Design review of the part built by this model. Coordinates are the model's own, in mm. Face numbers are marked on the shaded views. A direction names the side the tool comes from. Coordinates: 2 decimals unless noted, no trailing zeros. Loops run counter-clockwise (first coordinate to the right, second up) from the corner with the lowest first, then second, coordinate; pieces in that order, holes last. Notation, with made-up numbers: (43.25, -25.75) -> (87.25, -25.75) arc R23 cw to (87.25, 1.25) -> close; hole circle Ø8 at (7, 69.25). An arc over 180 degrees is marked (long way). Use one line per item in the form item = value. Start each with the question number.
1. Machinability: for the marked faces 1, 2, 3, 4 and 5, which of the approach directions +Z, -Z, +X, -X, +Y, -Y give a long, thin tool a straight path to every point of the face, cutting with its end or side? Answer none if there is none.
2. Consider section A-A (x = 51.75). State the section outline as (y, z) points.
3. The part is to be moulded in two halves that separate along Y. For the marked faces 6, 7 and 8, say which applies: released by +Y, released by -Y, zero draft, split by the parting line, or undercut.
4. For pin 1 (3.5 mm diameter, centred on y = 9.5, z = 30.09, fed in from +X); pin 2 (1.8 mm diameter, centred on y = 8, z = 0.5, fed in from +X); pin 3 (5 mm diameter, centred on y = 8.5, z = 32, fed in from +X), all flat-tipped, find the tip position at first contact; note any pin that passes through.
5. Consider section D-D (z = 13). State the section outline as (x, y) points, then the cut area to 3 significant figures.
6. Wall thickness on line 1 (Y direction, x = 55.5, z = 23); line 2 (Z direction, x = 40.5, y = 11.25); line 3 (X direction, y = 3.25, z = 16): over which ranges is each line inside the solid? List them lowest first. Write a range as from..to.
7. Consider section C-C (z = 29). State the section outline as (x, y) points.
8. Consider section B-B (y = 9.5). State the section outline as (x, z) points, then the cut area to 3 significant figures.
from build123d import *

# Parameters (mm, degrees)
SKETCH1_W           = 26
SKETCH1_H           = 37.2
BOSS_EXTRUDE1_DEPTH = 19
SKETCH2_W           = 20
SKETCH2_H           = 10
CUT_EXTRUDE1_DEPTH  = 77.929109018
SKETCH3_R           = 1.6
CUT_EXTRUDE2_DEPTH  = 76.699707134
CUT_EXTRUDE3_DEPTH  = 76.699707134
SKETCH7_W           = 22.2
SKETCH7_H           = 10
CUT_EXTRUDE6_DEPTH  = 45.240228818
SKETCH8_R           = 1.6
CUT_EXTRUDE7_DEPTH  = 45.240228818
CHAMFER1_SIZE       = 2
SKETCH9_R           = 2.9
CUT_EXTRUDE12_DEPTH = 2


with BuildPart() as part:
    # Sketch1 → Boss-Extrude1 (new body)
    with BuildSketch(Plane(origin=(0, 0, 0), x_dir=(1, 0, 0), z_dir=(0, 1, 0))):
        with Locations((51.600679674, -15.986093244)):
            Rectangle(SKETCH1_W, SKETCH1_H)
    extrude(amount=BOSS_EXTRUDE1_DEPTH)

    # Sketch2 → Cut-Extrude1 (cut, through all)
    with BuildSketch(Plane.XY.offset(34.586093244)):
        with Locations((54.600679674, 9.5)):
            Rectangle(SKETCH2_W, SKETCH2_H)
    extrude(amount=-CUT_EXTRUDE1_DEPTH, mode=Mode.SUBTRACT)

    # Sketch3 → Cut-Extrude2 (cut, through all)
    with BuildSketch(Plane.XZ):
        with Locations(Location((55.600679674, 15.986093244, 0), (0, 0, 270))):
            Circle(SKETCH3_R)
    extrude(amount=-CUT_EXTRUDE2_DEPTH, mode=Mode.SUBTRACT)

    # Sketch4 → Cut-Extrude3 (cut, through all)
    with BuildSketch(Plane.XZ):
        Polygon((64.600679674, 24.586093244), (54.600679674, 34.586093244), (64.600679674, 34.586093244), align=None)
        Polygon((64.600679674, 7.386093244), (54.600679674, -2.613906756), (64.600679674, -2.613906756), align=None)
    extrude(amount=-CUT_EXTRUDE3_DEPTH, mode=Mode.SUBTRACT)

    # Sketch7 → Cut-Extrude6 (cut, through all)
    with BuildSketch(Plane(origin=(44.600679674, 0, 0), x_dir=(0, 0, -1), z_dir=(1, 0, 0))):
        with Locations((-15.986093244, 9.5)):
            Rectangle(SKETCH7_W, SKETCH7_H)
    extrude(amount=-CUT_EXTRUDE6_DEPTH, mode=Mode.SUBTRACT)

    # Sketch8 → Cut-Extrude7 (cut, through all)
    with BuildSketch(Plane(origin=(44.600679674, 0, 0), x_dir=(0, 0, -1), z_dir=(1, 0, 0))):
        with Locations((-30.086093244, 9.5)):
            Circle(SKETCH8_R)
        with Locations((-1.886093244, 9.5)):
            Circle(SKETCH8_R)
    extrude(amount=-CUT_EXTRUDE7_DEPTH, mode=Mode.SUBTRACT)

    # Chamfer1
    chamfer1_edges = [part.edges().sort_by_distance(p)[0] for p in [
        (44.600679674, 4.5, 1.136093244),
        (44.600679674, 14.5, 1.136093244),
        (44.600679674, 14.5, 30.836093244),
        (44.600679674, 4.5, 30.836093244),
    ]]
    chamfer(chamfer1_edges, length=CHAMFER1_SIZE)

    # Sketch9 → Cut-Extrude12 (cut)
    with BuildSketch(Plane(origin=(44.600679674, 0, 0), x_dir=(0, 0, -1), z_dir=(1, 0, 0))):
        with Locations((-30.086093244, 9.5)):
            Circle(SKETCH9_R)
        with Locations((-1.886093244, 9.5)):
            Circle(SKETCH9_R)
    extrude(amount=-CUT_EXTRUDE12_DEPTH, mode=Mode.SUBTRACT)


solid = part.part
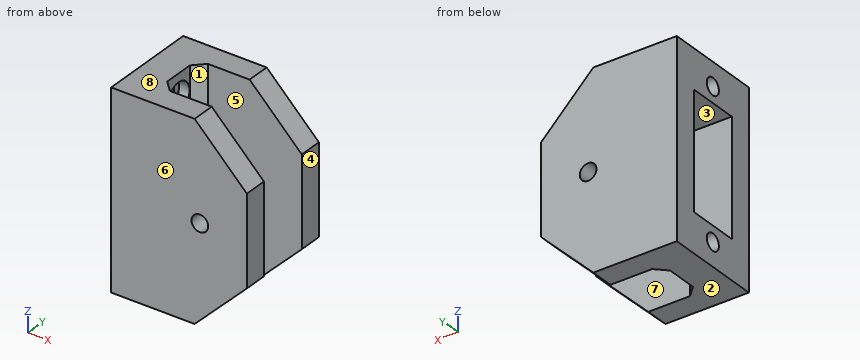
Geometry check:
q1.face_1 = +Z, -Z, +X
q1.face_2 = -Z, +X, -X, +Y, -Y
q1.face_3 = +X, -X
q1.face_4 = +Z, -Z, +X, +Y, -Y
q1.face_5 = +X
q2.outline = (0, -2.61) -> (4.5, -2.61) -> (4.5, 34.59) -> (0, 34.59) -> close; (14.5, -2.61) -> (19, -2.61) -> (19, 34.59) -> (14.5, 34.59) -> close
q3.face_6 = released by -Y
q3.face_7 = undercut
q3.face_8 = zero draft
q4.pin_1 = 42.6
q4.pin_2 = 44.6
q4.pin_3 = 45.1
q5.outline = (38.6, 0) -> (64.6, 0) -> (64.6, 4.5) -> (38.6, 4.5) -> close; (38.6, 14.5) -> (64.6, 14.5) -> (64.6, 19) -> (38.6, 19) -> close
q5.area = 234 mm²
q6.line_1 = 0..4.5, 14.5..19
q6.line_2 = -2.61..4.89, 27.09..34.59
q6.line_3 = 38.6..54, 57.2..64.6
q7.outline = (38.6, 0) -> (60.19, 0) -> (60.19, 4.5) -> (46.6, 4.5) -> (44.6, 6.5) -> (44.6, 6.81) -> (42.6, 6.81) -> (42.6, 8.33) -> (38.6, 8.33) -> close; (38.6, 10.67) -> (42.6, 10.67) -> (42.6, 12.19) -> (44.6, 12.19) -> (44.6, 12.5) -> (46.6, 14.5) -> (60.19, 14.5) -> (60.19, 19) -> (38.6, 19) -> close
q8.outline = (38.6, -2.61) -> (44.6, -2.61) -> (44.6, -1.01) -> (42.6, -1.01) -> (42.6, 0.29) -> (38.6, 0.29) -> close; (38.6, 3.49) -> (42.6, 3.49) -> (42.6, 4.79) -> (44.6, 4.79) -> (44.6, 4.89) -> (38.6, 4.89) -> close; (38.6, 27.09) -> (44.6, 27.09) -> (44.6, 27.19) -> (42.6, 27.19) -> (42.6, 28.49) -> (38.6, 28.49) -> close; (38.6, 31.69) -> (42.6, 31.69) -> (42.6, 32.99) -> (44.6, 32.99) -> (44.6, 34.59) -> (38.6, 34.59) -> close
q8.area = 41.2 mm²
